The model under review builds one solid part; all positions refer to its coordinate system, in mm. Coordinates: 2 decimals unless noted, no trailing zeros. Write each loop counter-clockwise with the first axis right and the second up, starting at its lowest first coordinate (ties: lowest second). Pieces come first, ordered by that corner, then holes. Notation, with made-up numbers: (-19.5, 83.5) - (21.5, 83.5) arc R23 ccw to (21.5, 102.5) - close; hole circle Ø5 at (-22, -25.5). An arc over 180 degrees is marked (long way). Put each result on its own line as item: value. Start each with the question number.
Item 1: To check wall thickness, follow L1, parallel to X at y = 10.75, z = 10.75; L2, parallel to Y at x = -4, z = 4.75; L3, parallel to Y at x = 4, z = 17.25. State the ranges of each line that lie inside material, in increasing order. Write a range as [from, to].
Item 2: Consider section B-B on z = 3.5. Give the boundary of the cut face in (x, y), then the cut area to 3 significant figures.
Item 3: For pin 1 (10 mm diameter, centred on x = 8.5, y = 5, fed in from -Z); pin 2 (12 mm diameter, centred on y = -1.5, z = 5, fed in from +X); pin 3 (4 mm diameter, centred on x = -2.5, z = 12.5, fed in from +Y), all flat-tipped, find the tip position at first contact; note any pin that passes through.
```python
from build123d import *

# Parameters (mm, degrees)
F1_DEPTH = 20
F2_SIZE  = 9.99999


# Not quite as in the source:
# - a fillet or chamfer is up to 0.001 mm smaller than in the source, because OpenCascade refuses the exact size


with BuildPart() as f1:
    # F0 (on Top) → F1 (new body)
    with BuildSketch(Plane.XY):
        Polygon((-5.9708582602, -14.4149269909), (5.9708582602, -14.4149269909), (11.5348123973, -8.8509728538), (14.4149269909, -3.8624680462), (14.4149269909, 3.8624680462), (11.5348123973, 8.8509728538), (5.9708582602, 14.4149269909), (-5.9708582602, 14.4149269909), (-11.5348123973, 8.8509728538), (-14.4149269909, 3.8624680462), (-14.4149269909, -3.8624680462), (-11.5348123973, -8.8509728538), align=None)
        Polygon((-14.4149269909, -5.9708582602), (-11.5348123973, -8.8509728538), (-14.4149269909, -3.8624680462), align=None)
        Polygon((-14.4149269909, 5.9708582602), (-14.4149269909, 3.8624680462), (-11.5348123973, 8.8509728538), align=None)
        Polygon((14.4149269909, -3.8624680462), (11.5348123973, -8.8509728538), (14.4149269909, -5.9708582602), align=None)
        Polygon((11.5348123973, 8.8509728538), (14.4149269909, 3.8624680462), (14.4149269909, 5.9708582602), align=None)
    extrude(amount=F1_DEPTH)

    # F2 (size 10 in the source; OpenCascade refuses exactly that, so slightly less here)
    f2_edges = [f1.edges().sort_by_distance(p)[0] for p in [
        (0, 14.414927, 20),
        (-10.192893, 10.192893, 20),
        (-14.414927, 0, 20),
        (-10.192893, -10.192893, 20),
        (0, -14.414927, 20),
        (10.192893, -10.192893, 20),
        (14.414927, 0, 20),
        (10.192893, 10.192893, 20),
        (0, 14.414927, 0),
        (-10.192893, 10.192893, 0),
        (-14.414927, 0, 0),
        (-10.192893, -10.192893, 0),
        (0, -14.414927, 0),
        (10.192893, -10.192893, 0),
        (14.414927, 0, 0),
        (10.192893, 10.192893, 0),
    ]]
    chamfer(f2_edges, length=F2_SIZE)


solid = f1.part
```
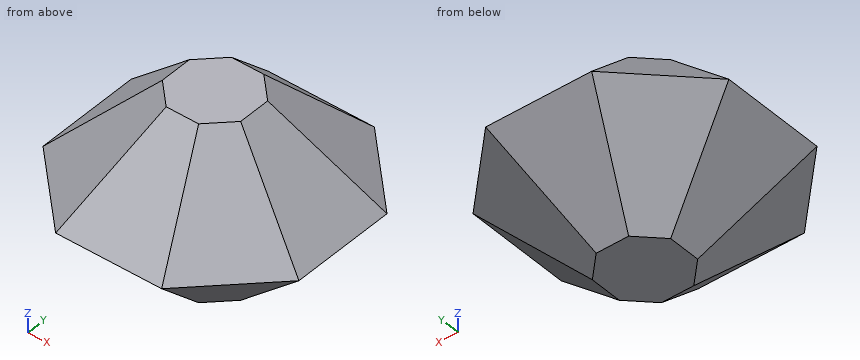
Report:
1. L1: [-8.58, 8.58]
1. L2: [-8.96, 8.96]
1. L3: [-6.13, 6.13]
2. outline: (-7.91, -3.28) - (-3.28, -7.91) - (3.28, -7.91) - (7.91, -3.28) - (7.91, 3.28) - (3.28, 7.91) - (-3.28, 7.91) - (-7.91, 3.28) - close
2. area: 208 mm²
3. pin 1: z = 0.16
3. pin 2: x = 14.41
3. pin 3: y = 13.91
